The drawing under review shows one solid part. Ordinate dimensions are in mm from its lowest x, y, z. A direction names the side the tool comes from. Coordinates: 2 decimals unless noted, no trailing zeros. Order: outer loops, then holes, each group sorted by start corner. A loop starts at its lowest first (then second) coordinate and runs counter-clockwise, first axis right, second up. Notation, with made-up numbers: (-5, 23) -> (31, 23) arc R21 cw to (31, 38) -> close; hole circle Ø3 at (25, 85.5). An arc over 180 degrees is marked (long way). Write item = value, one per line.
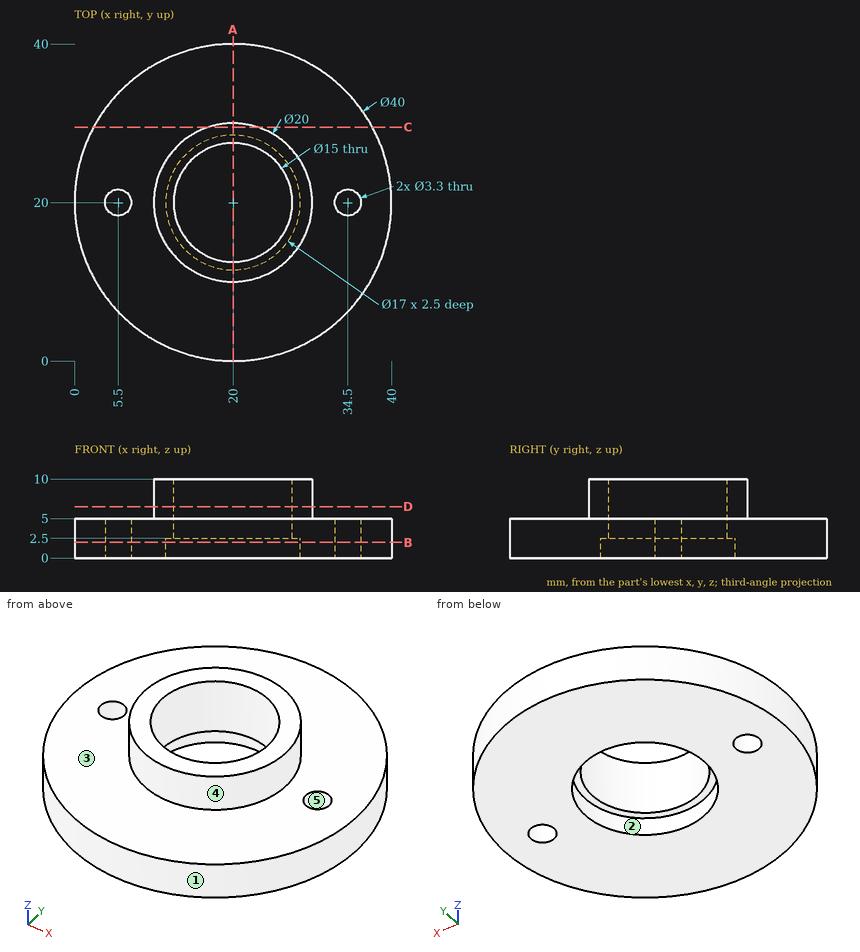
(1) Insertion check: pin 1 (4 mm diameter, centred on y = 28, z = 4, fed in from -X); pin 2 (2.5 mm diameter, centred on x = 5.5, y = 20, fed in from -Z); pin 3 (2 mm diameter, centred on y = 23, z = 4.5, fed in from +X); pin 4 (5.5 mm diameter, centred on x = 34.5, y = 20, fed in from +Z). Each pin has a flat end and moves straight along its axis. Give the tip position at first contact, or say it passes through.
Report:
pin_1 = 0.92
pin_2 = through
pin_3 = 39.9
pin_4 = 5
(2) We need section C-C (y = 29.5). Write out the cut boundary in (x, z).
Report:
outline = (2.4, 0) -> (37.6, 0) -> (37.6, 5) -> (23.12, 5) -> (23.12, 10) -> (16.88, 10) -> (16.88, 5) -> (2.4, 5) -> close
(3) For L1, parallel to X at y = 20, z = 6.25; L2, parallel to X at y = 19.5, z = 3.5, list the stretches that pass through material, from the lowest coordinate up.
Report:
L1 = 10 to 12.5, 27.5 to 30
L2 = 0.01 to 3.93, 7.07 to 12.52, 27.48 to 32.93, 36.07 to 39.99
(4) For the marked faces 4 and 5, list the 3-axis set-ups (+Z, -Z, +X, -X, +Y, -Y) from which the entire face can be reached by the end or side of a thin tool; tool diameter is ignored.
Report:
face_4 = +Z
face_5 = +Z, -Z
(5) We need section A-A (x = 20). Write out the cut boundary in (y, z), and give its area (3 significant figures).
Report:
outline = (0, 0) -> (11.5, 0) -> (11.5, 2.5) -> (12.5, 2.5) -> (12.5, 10) -> (10, 10) -> (10, 5) -> (0, 5) -> close; (27.5, 2.5) -> (28.5, 2.5) -> (28.5, 0) -> (40, 0) -> (40, 5) -> (30, 5) -> (30, 10) -> (27.5, 10) -> close
area = 145 mm²
(6) The part is to be moulded in two halves that separate along Y. For the marked faces 1, 2 and 3, say which applies: released by +Y, released by -Y, zero draft, split by the parting line, or undercut.
Report:
face_1 = split by the parting line
face_2 = undercut
face_3 = zero draft
(7) We need section B-B (z = 2). Write out the cut boundary in (x, y).
Report:
outline = circle Ø40 at (20, 20); hole circle Ø3.3 at (5.5, 20); hole circle Ø17 at (20, 20); hole circle Ø3.3 at (34.5, 20)
(8) We need section D-D (z = 6.5). Write out the cut boundary in (x, y).
Report:
outline = circle Ø20 at (20, 20); hole circle Ø15 at (20, 20)
